Build history of the part. All positions in model axes, mm. A direction names the side the tool comes from. Coordinates: 2 decimals unless noted, no trailing zeros. One line per item, written item: value.
from build123d import *

# Parameters (mm, degrees)
FILLET1_R          = 0.254
CHAMFER1_SIZE      = 0.254
SKETCH2_W          = 4.146231659
SKETCH2_H          = 2.159
CUT_EXTRUDE1_DEPTH = 50.872125446


with BuildPart() as part:
    # Sketch1 → Revolve1 (revolve)
    with BuildSketch(Plane.XY, mode=Mode.PRIVATE) as revolve1_sk:
        Polygon((35.2425, 0), (35.2425, 1.778), (31.877, 1.778), (31.877, 1.016), (31.115, 1.016), (31.115, 0), align=None)
    revolve(revolve1_sk.sketch.rotate(Axis((0, 0, 0), (0, 1, 0)), 90), axis=Axis((0, 0, 0), (0, 1, 0)))

    # Fillet1
    fillet1_edges = [part.edges().sort_by_distance(p)[0] for p in [
        (0, 1.016, 31.877),
    ]]
    fillet(fillet1_edges, radius=FILLET1_R)

    # Chamfer1
    chamfer1_edges = [part.edges().sort_by_distance(p)[0] for p in [
        (0, 1.778, 35.2425),
        (0, 0, 35.2425),
    ]]
    chamfer(chamfer1_edges, length=CHAMFER1_SIZE)

    # Sketch2 → Cut-Extrude1 (cut, through all)
    with BuildSketch(Plane(origin=(0, 1.778, 0), x_dir=(1, 0, 0), z_dir=(0, 1, 0))):
        with Locations((-33.169384171, 0)):
            Rectangle(SKETCH2_W, SKETCH2_H)
    extrude(amount=-CUT_EXTRUDE1_DEPTH, mode=Mode.SUBTRACT)


solid = part.part
1. Two-plate mould, pull along Z, no slides. Class faces 1 (the face through (7.6, 1.778, 31.3)), 2 (the face through (-33, 1, -1.08)): pulls with the +Z half, pulls with the -Z half, needs draft (parallel to the pull), parting line crosses it, or undercut.
Values found:
face 1: needs draft
face 2: undercut
2. Probe line 1 along X through (y, z) = (1.45, 0); line 2 along X through (y, z) = (0.35, 0) (1 decimal); line 3 along Z through (x, y) = (25, 0.2). List the from-to ranges inside material, lowest first.
Values found:
line 1: x = 31.88 to 35.24
line 2: x = 31.1 to 35.2
line 3: z = -24.76 to -18.52, 18.52 to 24.76
3. 3-axis set-ups, long thin cutter, end or side, ignore diameter. For faces 3 (the face through (28, 1.016, -14)), 4 (the face through (-33, 1, 1.08)), 5 (the face through (-31.2, 0, -2.8)): which of +Z, -Z, +X, -X, +Y, -Y reach the whole face in a straight line?
Values found:
face 3: +Y
face 4: -X, +Y, -Y
face 5: +Z, -Z, +X, -X, -Y
